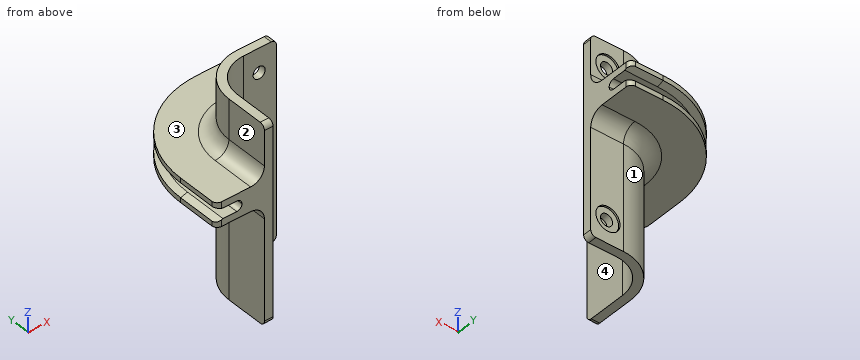
```python
from build123d import *

# Parameters (mm, degrees)
F1_DEPTH  = 40
F3_DEPTH  = 6.5
F4_DEPTH  = 14
F5_R      = 3.5
F5_R_2    = 1.75
F6_DEPTH  = 0.5
F7_DEPTH  = 25
F8_DEPTH  = 17
F9_R      = 1.75
F10_DEPTH = 3
F9_R_2    = 3.5
F11_DEPTH = 0.5
F12_W     = 12.5
F12_H     = 3
F13_DEPTH = 6.5
F12_H_2   = 2
F14_DEPTH = 14
F15_ANGLE = 90
F16_R     = 4
F17_SIZE2 = 2
F17_SIZE  = 0.6
F18_SIZE2 = 0.6
F18_SIZE  = 2
F19_R     = 1.49999


# Not quite as in the source:
# - a fillet or chamfer is up to 0.001 mm smaller than in the source, because OpenCascade refuses the exact size


with BuildPart() as f1:
    # F0 (on Top) → F1 (new body)
    with BuildSketch(Plane.XY):
        with BuildLine():
            ThreePointArc((-10, 0), (-7.0710678119, 7.0710678119), (0, 10))
            Line((0, 10), (9.5, 10))
            Line((9.5, 10), (9.5, 12.5))
            Line((9.5, 12.5), (0, 12.5))
            ThreePointArc((0, 12.5), (-8.8388347648, 8.8388347648), (-12.5, 0))
            Line((-12.5, 0), (-12.5, -12.5))
            Line((-12.5, -12.5), (-10, -12.5))
            Line((-10, -12.5), (-10, 0))
        make_face()
    extrude(amount=F1_DEPTH)

    # F2 (on face) → F3 (join)
    with BuildSketch(Plane(origin=(0, 12.5, 0), x_dir=(-1, 0, 0), z_dir=(0, 1, 0))):
        Polygon((-5.7388888672, 22.5), (-9.5, 22.5), (-9.5, 19.5), (-5.7327155955, 19.5), (0, 19.5), (0, 22.5), align=None)
    extrude(amount=F3_DEPTH)

    # F2 (on face) → F4 (join)
    with BuildSketch(Plane(origin=(0, 12.5, 0), x_dir=(-1, 0, 0), z_dir=(0, 1, 0))):
        Polygon((-5.7188421488, 24.5), (-9.5, 24.5), (-9.5, 22.5), (-5.7388888672, 22.5), (0, 22.5), (0, 24.5), align=None)
        Polygon((-5.7327155955, 19.5), (-9.5, 19.5), (-9.5, 17.5), (-5.7445626465, 17.5), (0, 17.5), (0, 19.5), align=None)
    extrude(amount=F4_DEPTH)

    # F5 (on face) → F6 (cut)
    with BuildSketch(Plane(origin=(0, 12.5, 0), x_dir=(-1, 0, 0), z_dir=(0, 1, 0))):
        with Locations((-4.5, 33)):
            Circle(F5_R)
        with Locations((-4.5, 33)):
            Circle(F5_R_2, mode=Mode.SUBTRACT)
    extrude(amount=-F6_DEPTH, mode=Mode.SUBTRACT)

    # F5 (on face) → F7 (cut)
    with BuildSketch(Plane(origin=(0, 12.5, 0), x_dir=(-1, 0, 0), z_dir=(0, 1, 0))):
        with Locations((-4.5, 33)):
            Circle(F5_R_2)
    extrude(amount=-F7_DEPTH, mode=Mode.SUBTRACT)

    # F8 (add): a face of the model
    f8_faces = [f1.faces().sort_by_distance(p)[0] for p in [
        (-7.3065460487, 7.3065460487, 0),
    ]]
    extrude(f8_faces, amount=F8_DEPTH)

    # F9 (on face) → F10 (cut)
    with BuildSketch(Plane(origin=(0, 12.5, 0), x_dir=(-1, 0, 0), z_dir=(0, 1, 0))):
        with Locations((-4.5, -10)):
            Circle(F9_R)
    extrude(amount=-F10_DEPTH, mode=Mode.SUBTRACT)

    # F9 (on face) → F11 (cut)
    with BuildSketch(Plane(origin=(0, 12.5, 0), x_dir=(-1, 0, 0), z_dir=(0, 1, 0))):
        with Locations((-4.5, -10)):
            Circle(F9_R_2)
        with Locations((-4.5, -10)):
            Circle(F9_R, mode=Mode.SUBTRACT)
    extrude(amount=-F11_DEPTH, mode=Mode.SUBTRACT)

    # F12 (on face) → F13 (join)
    with BuildSketch(Plane(origin=(-12.5, 0, 0), x_dir=(0, -1, 0), z_dir=(-1, 0, 0))):
        with Locations((6.25, 21)):
            Rectangle(F12_W, F12_H)
    extrude(amount=F13_DEPTH)

    # F12 (on face) → F14 (join)
    with BuildSketch(Plane(origin=(-12.5, 0, 0), x_dir=(0, -1, 0), z_dir=(-1, 0, 0))):
        with Locations((6.25, 23.5)):
            Rectangle(F12_W, F12_H_2)
        with Locations((6.25, 18.5)):
            Rectangle(F12_W, F12_H_2)
    extrude(amount=F14_DEPTH)

    # F14_face (on face) → F15 (revolve)
    with BuildSketch(Plane(origin=(-18.5314569536, 0, 21), x_dir=(-1, 0, 0), z_dir=(0, 1, 0))):
        Polygon((7.9685430464, -1.5), (0.4685430464, -1.5), (0.4685430464, 1.5), (7.9685430464, 1.5), (7.9685430464, 3.5), (-6.0314569536, 3.5), (-6.0314569536, -3.5), (7.9685430464, -3.5), align=None)
    revolve(axis=Axis((0, 0, 0), (0, 0, -1)), revolution_arc=F15_ANGLE)

    # F16
    f16_edges = [f1.edges().sort_by_distance(p)[0] for p in [
        (-8.838835, 8.838835, 17.5),
        (-8.838835, 8.838835, 24.5),
    ]]
    fillet(f16_edges, radius=F16_R)

    # F17
    f17_edges = [f1.edges().sort_by_distance(p)[0] for p in [
        (-26.5, -6.25, 19.5),
    ]]
    f17_side = f1.faces().sort_by_distance((-26.5, -6.25, 18.5))[0]
    chamfer(f17_edges, length=F17_SIZE, length2=F17_SIZE2, reference=f17_side)

    # F18
    f18_edges = [f1.edges().sort_by_distance(p)[0] for p in [
        (-26.5, -6.25, 22.5),
    ]]
    f18_side = f1.faces().sort_by_distance((-19.530754, -6.25, 22.5))[0]
    chamfer(f18_edges, length=F18_SIZE, length2=F18_SIZE2, reference=f18_side)

    # F19 (radius 1.5 in the source; OpenCascade refuses exactly that, so slightly less here)
    f19_edges = [f1.edges().sort_by_distance(p)[0] for p in [
        (-13.435029, 13.435029, 19.5),
        (-13.435029, 13.435029, 22.5),
        (9.5, 26.5, 23.8),
        (9.5, 26.5, 18.2),
        (-26.5, -12.5, 18.2),
        (-26.5, -12.5, 23.8),
        (-11.25, -12.5, 40),
        (9.5, 11.25, 40),
        (9.5, 11.25, -17),
        (-11.25, -12.5, -17),
    ]]
    fillet(f19_edges, radius=F19_R)


solid = f1.part
```
Geometry check sheet. Reference: the model listing, model coordinates, mm. Face numbers are marked on the shaded views. A direction names the side the tool comes from. Give positions to 0.01 mm unless a question says otherwise; leave off trailing zeros. Loops run counter-clockwise (first coordinate to the right, second up) from the corner with the lowest first, then second, coordinate; pieces in that order, holes last. Notation, with made-up numbers: M 68.5,20.25 L 106.5,20.25 A16 ccw 106.5,36.25 Z; hole C -16,83.5 d3. An arc over 180 degrees is marked long. Write item = value, one per line.
(1) Material ranges on line 1 (Z direction, x = 4.5, y = 12.15); line 2 (Z direction, x = 4.5, y = 11.15); line 3 (Z direction, x = -11, y = 18.5), recorded low to high. Write a range as [from, to].
Answer below:
line_1 = [-17, -13.5], [-6.5, 29.5], [36.5, 40]
line_2 = [-17, -11.75], [-8.25, 31.25], [34.75, 40]
line_3 = [17.5, 19.5], [22.5, 24.5]
(2) Gauge pin test, flat ends, axial feed: pin 1 Ø4 at (y, z) = (21.5, 27.5) entering from +X; pin 2 Ø11 at (x, y) = (-16.5, 12) entering from -Z; pin 3 Ø3 at (x, y) = (-8.5, 3) entering from +Z; pin 4 Ø7.5 at (x, z) = (5, -9) entering from +Y. Record the tip position at first contact, or that the pin passes through.
Answer below:
pin_1 = through
pin_2 = 17.17
pin_3 = 40
pin_4 = 12.5
(3) Tool access check on the marked faces 1, 2, 3 and 4. Record the directions out of +Z, -Z, +X, -X, +Y, -Y that give a thin tool (end or side, any length) a straight path to the whole face; none if there is none.
Answer below:
face_1 = -Z, -X, +Y
face_2 = +Z, -X, +Y, -Y
face_3 = +Z, -X, +Y
face_4 = +Z, -Z, +X, -Y
(4) Sectioned sample at B-B, the plane z = 33. Record the cut outline in (x, y).
Answer below:
outline = M -12.5,-12.5 L -10,-12.5 L -10,0 A10 cw 0,10 L 2.75,10 L 2.75,12 L 1,12 L 1,12.5 L 0,12.5 A12.5 ccw -12.5,0 Z; M 6.25,10 L 9.5,10 L 9.5,12.5 L 8,12.5 L 8,12 L 6.25,12 Z
(5) Sectioned sample at C-C, the plane z = 6. Record the cut outline in (x, y).
Answer below:
outline = M -12.5,-12.5 L -10,-12.5 L -10,0 A10 cw 0,10 L 9.5,10 L 9.5,12.5 L 0,12.5 A12.5 ccw -12.5,0 Z
(6) Sectioned sample at A-A, the plane x = 4.5. State how many separate pieces and enclosed holes the cut face has, plus the area to 3 significant figures.
Answer below:
separate_pieces = 3
enclosed_holes = 0
area = 204 mm2
